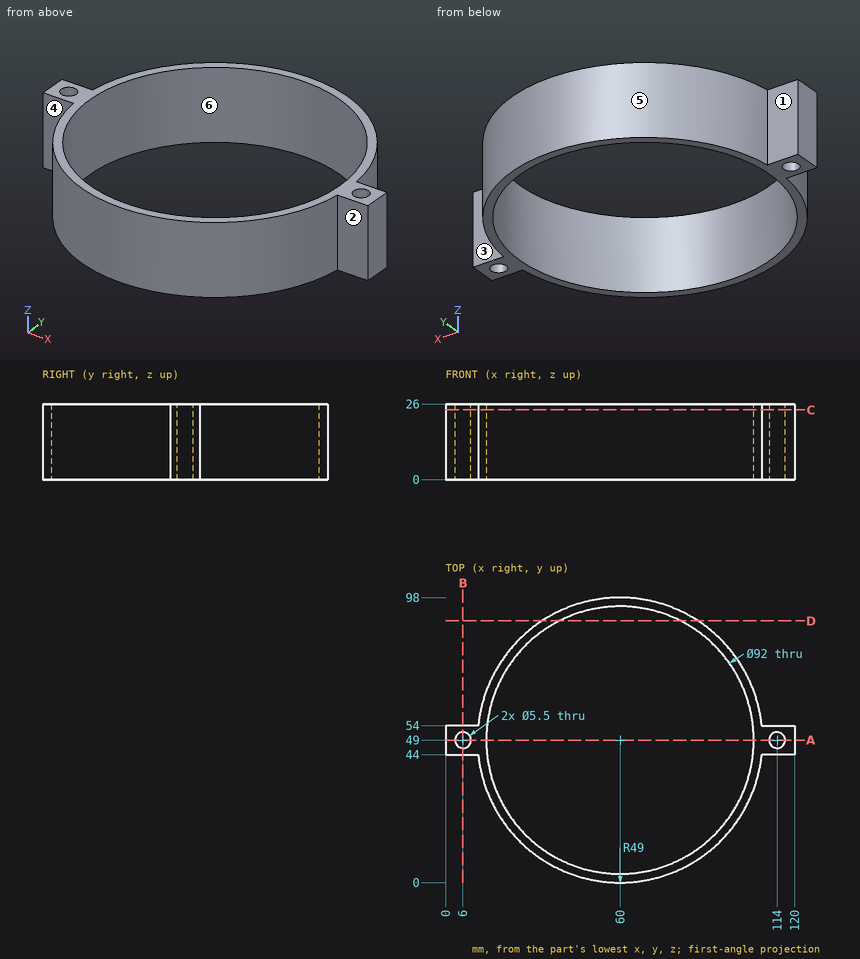
Study the drawing (mm; zero at the part's minimum x, y, z) and answer. A direction names the side the tool comes from. Give positions to 0.01 mm unless a question says otherwise; leave off trailing zeros. Write each loop counter-clockwise with the first axis right and the second up, starting at its lowest first coordinate (ties: lowest second). Pieces come first, ordered by that corner, then holes. Notation, with made-up numbers: (81.25, 69.25) -> (132.25, 69.25) arc R17 cw to (132.25, 89.25) -> close; hole circle Ø7 at (82.25, 19.25). An arc over 180 degrees is marked (long way). Write item = value, one per line.
Q1. Section B-B on x = 6 is taken. Determine the outline of the cut face in (y, z).
Computed values:
outline = (44, 0) -> (46.25, 0) -> (46.25, 26) -> (44, 26) -> close; (51.75, 0) -> (54, 0) -> (54, 26) -> (51.75, 26) -> close
Q2. Section C-C on z = 24 is taken. Determine the outline of the cut face in (x, y).
Computed values:
outline = (0, 44) -> (11.26, 44) arc R49 ccw to (108.74, 44) -> (120, 44) -> (120, 54) -> (108.74, 54) arc R49 ccw to (11.26, 54) -> (0, 54) -> close; hole circle Ø5.5 at (6, 49); hole circle Ø92 at (60, 49); hole circle Ø5.5 at (114, 49)
Q3. For a pull along X with two mould halves and no side action, classify the marked faces 4, 5 and 6 as pulls with the +X half, pulls with the -X half, needs draft (parallel to the pull), parting line crosses it, or undercut.
Computed values:
face_4 = needs draft
face_5 = parting line crosses it
face_6 = undercut
Q4. Section A-A on y = 49 is taken. Determine the outline of the cut face in (x, z).
Computed values:
outline = (0, 0) -> (3.25, 0) -> (3.25, 26) -> (0, 26) -> close; (8.75, 0) -> (14, 0) -> (14, 26) -> (8.75, 26) -> close; (106, 0) -> (111.25, 0) -> (111.25, 26) -> (106, 26) -> close; (116.75, 0) -> (120, 0) -> (120, 26) -> (116.75, 26) -> close
Q5. Section D-D on y = 90 is taken. Determine the outline of the cut face in (x, z), and give its area (3 significant figures).
Computed values:
outline = (33.17, 0) -> (39.14, 0) -> (39.14, 26) -> (33.17, 26) -> close; (80.86, 0) -> (86.83, 0) -> (86.83, 26) -> (80.86, 26) -> close
area = 311 mm^2
Q6. A tool of negligible diameter and unlimited length cuts with its end or side. For the marked faces 1, 2 and 3, from which of +Z, -Z, +X, -X, +Y, -Y can it reach the whole face along a straight path? Write none if from no direction.
Computed values:
face_1 = +Z, -Z, -X, +Y
face_2 = +Z, -Z, +X, -Y
face_3 = +Z, -Z, +X, +Y
Q7. Flat-ended cylindrical pins translate along their axes: pin 1 Ø3.5 at (x, z) = (4, 16) entering from -Y; pin 2 Ø2 at (x, z) = (40, 3) entering from +Y; pin 3 Ø9 at (x, z) = (116.5, 15) entering from +Y. Find the tip coordinate at first contact, or state that the pin passes through.
Computed values:
pin_1 = 44
pin_2 = 94.17
pin_3 = 54
Q8. Consider line 1 along Y through (x, z) = (6, 14.25); line 2 along X through (y, z) = (51.5, 6.75); line 3 along X through (y, z) = (48, 2.5). Determine where each line is inside the solid, lowest interval first.
Computed values:
line_1 = 44 to 46.25, 51.75 to 54
line_2 = 0 to 4.85, 7.15 to 14.07, 105.93 to 112.85, 115.15 to 120
line_3 = 0 to 3.44, 8.56 to 14.01, 105.99 to 111.44, 116.56 to 120
